Design review of the part built by this model. Coordinates are the model's own, in mm. Face numbers are marked on the shaded views. A direction names the side the tool comes from. Round coordinates to 2 decimals unless told otherwise and drop trailing zeros. Loops run counter-clockwise (first coordinate to the right, second up) from the corner with the lowest first, then second, coordinate; pieces in that order, holes last. Notation, with made-up numbers: M 76.5,30 L 130.5,30 A18 ccw 130.5,65 Z; hole C 16.5,32.5 d2. An arc over 180 degrees is marked long. Use a Markdown table: item, result.
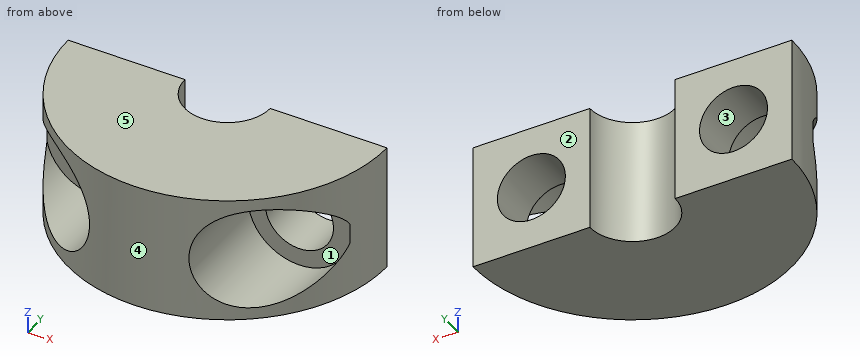
from build123d import *

# Parameters (mm, degrees)
BOSS_EXTRUDE1_DEPTH      = 6
BOSS_EXTRUDE1_DEPTH_BACK = 6


with BuildPart() as part:
    # Sketch1 → Boss-Extrude1 (new body, two sides)
    with BuildSketch(Plane.XY) as boss_extrude1_sk:
        with BuildLine():
            Line((15.1765, 0), (4.064, 0))
            ThreePointArc((4.064, 0), (0, -4.064), (-4.064, 0))
            Line((-4.064, 0), (-15.1765, 0))
            ThreePointArc((-15.1765, 0), (0, -15.1765), (15.1765, 0))
        make_face()
    extrude(amount=BOSS_EXTRUDE1_DEPTH)
    extrude(boss_extrude1_sk.sketch, amount=-BOSS_EXTRUDE1_DEPTH_BACK)

    # Sketch2 → Cut-Revolve1 (revolve, cut)
    with BuildSketch(Plane.XY):
        Polygon((-9.62025, 0), (-6.38175, 0), (-6.38175, -4.7625), (-4.73075, -4.7625), (-4.73075, -14.4203383), (-9.62025, -14.4203383), align=None)
    cut_revolve1 = revolve(axis=Axis((-9.62025, -14.4203383, 0), (0, 1, 0)), mode=Mode.SUBTRACT)

    # Mirror1: Cut-Revolve1 across plane
    add(cut_revolve1.mirror(Plane(origin=(0, 0, 0), x_dir=(0, 0, 1), z_dir=(1, 0, 0))), mode=Mode.SUBTRACT)


solid = part.part
1. Take a section at C-C on x = 10.5. Give the boundary of the cut face in (y, z).
Check values:
| item | result |
|---|---|
| outline | M -10.96,-6 L 0,-6 L 0,-3.12 L -4.76,-3.12 L -4.76,-4.81 L -10.96,-4.81 Z; M -10.96,4.81 L -4.76,4.81 L -4.76,3.12 L 0,3.12 L 0,6 L -10.96,6 Z |
2. The part is to be moulded in two halves that separate along X. For the marked faces 3, 4 and 5, say which applies: pulls with the +X half, pulls with the -X half, needs draft (parallel to the pull), parting line crosses it, or undercut.
Check values:
| item | result |
|---|---|
| face 3 | undercut |
| face 4 | parting line crosses it |
| face 5 | needs draft |
3. Take a section at D-D on y = -6. Give the boundary of the cut face in (x, z), and give its area (3 significant figures).
Check values:
| item | result |
|---|---|
| outline | M -13.94,-6 L 13.94,-6 L 13.94,-2.29 A4.89 cw long 13.94,2.29 L 13.94,6 L -13.94,6 L -13.94,2.29 A4.89 cw long -13.94,-2.29 Z |
| area | 188 mm² |
4. Take a section at A-A on z = 0. Give the boundary of the cut face in (x, y).
Check values:
| item | result |
|---|---|
| outline | M -15.18,0 A15.18 ccw -14.41,-4.76 L -12.86,-4.76 L -12.86,0 Z; M -6.38,-4.76 L -4.73,-4.76 L -4.73,-14.42 A15.18 ccw 4.73,-14.42 L 4.73,-4.76 L 6.38,-4.76 L 6.38,0 L 4.06,0 A4.06 cw -4.06,0 L -6.38,0 Z; M 12.86,-4.76 L 14.41,-4.76 A15.18 ccw 15.18,0 L 12.86,0 Z |
5. Insertion check: pin 1 (4 mm diameter, centred on x = 9.5, z = 2.5, fed in from -Y); pin 2 (3 mm diameter, centred on y = -2.5, z = -2.5, fed in from +X); pin 3 (1 mm diameter, centred on y = -8.5, z = -2.5, fed in from +X). Each pin has a flat end and moves straight along its axis. Give the tip position at first contact, or say it passes through.
Check values:
| item | result |
|---|---|
| pin 1 | stops at y = -4.76 |
| pin 2 | stops at x = 15.14 |
| pin 3 | stops at x = 5.76 |
6. Take a section at B-B on y = -2. Give the boundary of the cut face in (x, z), and give its area (3 significant figures).
Check values:
| item | result |
|---|---|
| outline | M -15.04,-6 L -3.54,-6 L -3.54,6 L -15.04,6 Z; M 3.54,-6 L 15.04,-6 L 15.04,6 L 3.54,6 Z; hole C -9.62,0 d6.48; hole C 9.62,0 d6.48 |
| area | 210 mm² |
7. Machinability: for the marked faces 1 and 2, which of the approach directions +Z, -Z, +X, -X, +Y, -Y give a long, thin tool a straight path to every point of the face, cutting with its end or side? Answer none if there is none.
Check values:
| item | result |
|---|---|
| face 1 | -Y |
| face 2 | +Z, -Z, +X, -X, +Y |
8. Wall thickness on line 1 along X through (y, z) = (-5.5, 3.75); line 2 along X through (y, z) = (-3.5, -2.25); line 3 along Y through (x, z) = (11, 3.25): over which ranges is each line inside the solid? List them lowest first. Write a range as from..to.
Check values:
| item | result |
|---|---|
| line 1 | x = -14.14..-12.76, -6.48..6.48, 12.76..14.14 |
| line 2 | x = -14.77..-11.95, -7.29..-2.07, 2.07..7.29, 11.95..14.77 |
| line 3 | y = -4.76..0 |
